Read the model definition and answer for the solid it produces. Units are mm, in the model's axes. A direction names the side the tool comes from. Give positions to 0.01 mm unless a question says otherwise; leave off trailing zeros. Order: outer loops, then holes, each group sorted by start corner. A loop starts at its lowest first (then second) coordinate and runs counter-clockwise, first axis right, second up. Notation, with made-up numbers: M 79.25,89 L 96.25,89 A6 ccw 96.25,95 Z; hole C 31,62.5 d4. An arc over 180 degrees is marked long. Write item = value, one per line. Start each with the question number.
Autodesk Inventor part; units mm, degrees
ref_plane "YZ Plane" through (0, 0, 0) normal (1, 0, 0) x (0, 1, 0)
ref_plane "XZ Plane" through (0, 0, 0) normal (0, 1, 0) x (-1, 0, 0)
ref_plane "XY Plane" through (0, 0, 0) normal (0, 0, 1) x (1, 0, 0)
sketch "Sketch1" plane through (0, 0, 0) normal (0, 0, 1) x (1, 0, 0)
  line L0 (-100, 0) -> (-100, 70)
  line L1 (-90, 80) -> (90, 80)
  line L2 (100, 70) -> (100, 0)
  arc A0 (-90, 80) -> (-100, 70) centre (-90, 70) ccw
  arc A1 (100, 70) -> (90, 80) centre (90, 70) ccw
  line L3 (-110, 0) -> (-110, 70)
  arc A2 (-90, 90) -> (-110, 70) centre (-90, 70) ccw
  arc A3 (110, 70) -> (90, 90) centre (90, 70) ccw
  line L4 (110, 70) -> (110, 0)
  line L5 (100, 0) -> (110, 0)
  line L6 (-100, 0) -> (-110, 0)
  line L7 (-90, 90) -> (-90, 100)
  line L8 (90, 90) -> (90, 100)
  line L9 (-50, 100) -> (-50, 117.5)
  line L10 (50, 100) -> (50, 117.5)
  line L11 (-18.114, 117.5) -> (0, 110)
  line L12 (0, 110) -> (18.114, 117.5)
  line L13 (-50, 117.5) -> (-18.114, 117.5)
  line L14 (18.114, 117.5) -> (50, 117.5)
  line L15 (-90, 100) -> (-50, 100)
  line L16 (50, 100) -> (90, 100)
  point P0 (0, 0)
  dimension "d0" = 100
  dimension "d1" = 100
  dimension "d2" = 80
  dimension "d4" = 10
  dimension "d5" = 10
  dimension "d24" = 10
  dimension "d25" = 50
  dimension "d26" = 50
  dimension "d31" = 31.886
  dimension "d33" = 50
  dimension "d37" = 10
  dimension "d38" = 20
  dimension "d39" = 20
  dimension "d40" = 17.5
  dimension "d41" = 17.5
extrude "Extrusion1" add sketch "Sketch1" against normal blind 150
sketch "Sketch4" plane through (-90, 100, 0) normal (0, 1, 0) x (1, 0, 0)
  circle A0 centre (20, 75) radius 8
  circle A1 centre (160, 75) radius 8
  line L0 (0, 0) -> (0, 150)
  line L1 (40, 0) -> (0, 0)
  line L2 (180, 0) -> (180, 150)
  line L3 (180, 0) -> (140, 0)
  point P0 (90, 0)
  dimension "d42" = 16
  dimension "d43" = 20
  dimension "d44" = 20
  dimension "d45" = 75
  dimension "d46" = 75
extrude "Extrusion4" cut sketch "Sketch4" against normal blind 50
equation "\"d33\" = d25"
equation "\"d39\" = d38"
equation "\"d41\" = d40"
equation "\"d44\" = d43"
equation "\"d46\" = d45"
equation "\"d36\" = d34"
properties part number "Base soporte tubos"
1) For a pull along X with two mould halves and no side action, classify faces 5 (the face through (-71.041, 90.14, -82.932)), 6 (the face through (61, 100, -74)), 7 (the face through (-103.986, 84.297, -73.95)) as pulls with the +X half, pulls with the -X half, needs draft (parallel to the pull), parting line crosses it, or undercut.
2) Find section C-C on z = -75. Count the separate pieces of the cut face and the enclosed holes in it, plus the area to 3 significant figures.
3) Find section A-A on x = 70. Determine the outline of the cut face in (y, z).
4) Find section D-D on z = -124.5. Determine the outline of the cut face in (x, y).
5) Find the intervals of material crossed by probe 1 along X at (y, z) = (92, -75); probe 2 along Z at (x, y) = (70, 90.5); probe 3 along X at (y, z) = (69, -91.5), in increasing order. Write a range as [from, to].
6) For faces 1 (the face through (-100, 35, -74)), 2 (the face through (90, 95, -74)), 3 (the face through (-90, 95, -74)), 4 (the face through (-9.18, 113.8, -73.95)), determine the directions among +Z, -Z, +X, -X, +Y, -Y from which every point of the face is accessible in a straight line to the end or side of a thin tool.
7) Find section B-B on y = 27.5. Determine the outline of the cut face in (x, z).
8) Each of these flat-tipped pins is pushed along its axis until it touches: P1, Ø11, axis at y = 93.5, z = -45, coming from the +X side; P2, Ø5, axis at y = 93, z = -98, coming from the -X side; P3, Ø8, axis at x = 38, z = -30.5, coming from the -Y side; P4, Ø13, axis at x = 70, z = -75, coming from the +Y side. Where does it stop, or does it pass through?
Numbers:
q1.face_5 = undercut
q1.face_6 = needs draft
q1.face_7 = pulls with the -X half
q2.separate_pieces = 3
q2.enclosed_holes = 0
q2.area = 6,450 mm2
q3.outline = M 80,-150 L 100,-150 L 100,-83 L 80,-83 Z; M 80,-67 L 100,-67 L 100,0 L 80,0 Z
q4.outline = M -110,0 L -100,0 L -100,70 A10 cw -90,80 L 90,80 A10 cw 100,70 L 100,0 L 110,0 L 110,70 A20 ccw 90,90 L 90,100 L 50,100 L 50,117.5 L 18.11,117.5 L 0,110 L -18.11,117.5 L -50,117.5 L -50,100 L -90,100 L -90,90 A20 ccw -110,70 Z
q5.probe_1 = [-90, -78], [-62, 62], [78, 90]
q5.probe_2 = [-150, -83], [-67, 0]
q5.probe_3 = [-110, -100], [100, 110]
q6.face_1 = +Z, -Z, -Y
q6.face_2 = +Z, -Z, +X, +Y
q6.face_3 = +Z, -Z, -X, +Y
q6.face_4 = +Z, -Z, +Y
q7.outline = M -110,-150 L -100,-150 L -100,0 L -110,0 Z; M 100,-150 L 110,-150 L 110,0 L 100,0 Z
q8.P1 = 98.72
q8.P2 = -90
q8.P3 = 80
q8.P4 = through
